Geometry check sheet. Reference: the model listing, model coordinates, mm. Give positions to 0.01 mm unless a question says otherwise; leave off trailing zeros. Write each loop counter-clockwise with the first axis right and the second up, starting at its lowest first coordinate (ties: lowest second). Pieces come first, ordered by that corner, then holes. Notation, with made-up numbers: (36, 86.5) -> (66, 86.5) arc R18 ccw to (66, 114.5) -> close; hole circle Ø3 at (86, 73.5). An arc over 180 degrees is marked (long way). One line per item, written item: value.
from build123d import *

# Parameters (mm, degrees)
ESQUISSE1_R        = 11
ESQUISSE1_R_2      = 1.65
ESQUISSE1_R_3      = 3
BOSS_EXTRU_1_DEPTH = 4
CHANFREIN1_SIZE    = 0.5


with BuildPart() as part:
    # Esquisse1 → Boss.-Extru.1 (new body)
    with BuildSketch(Plane(origin=(0, 0, 0), x_dir=(1, 0, 0), z_dir=(0, 1, 0))):
        with Locations(Location((0, 0, 0), (0, 0, 270))):
            Circle(ESQUISSE1_R)
        with Locations(Location((0, 7, 0), (0, 0, 270))):
            Circle(ESQUISSE1_R_2, mode=Mode.SUBTRACT)
        with Locations(Location((7, 0, 0), (0, 0, 270))):
            Circle(ESQUISSE1_R_2, mode=Mode.SUBTRACT)
        with Locations(Location((0, -7, 0), (0, 0, 270))):
            Circle(ESQUISSE1_R_2, mode=Mode.SUBTRACT)
        with Locations(Location((-7, 0, 0), (0, 0, 270))):
            Circle(ESQUISSE1_R_2, mode=Mode.SUBTRACT)
        with Locations(Location((0, 0, 0), (0, 0, 270))):
            Circle(ESQUISSE1_R_3, mode=Mode.SUBTRACT)
    extrude(amount=BOSS_EXTRU_1_DEPTH)

    # Chanfrein1
    chanfrein1_edges = [part.edges().sort_by_distance(p)[0] for p in [
        (0, 0, -11),
        (0, 4, -11),
    ]]
    chamfer(chanfrein1_edges, length=CHANFREIN1_SIZE)


solid = part.part
1) Sectioned sample at B-B on z = 0. Record the cut outline in (x, y).
Verdict:
outline: (-11, 0.5) -> (-10.5, 0) -> (-8.65, 0) -> (-8.65, 4) -> (-10.5, 4) -> (-11, 3.5) -> close; (-5.35, 0) -> (-3, 0) -> (-3, 4) -> (-5.35, 4) -> close; (3, 0) -> (5.35, 0) -> (5.35, 4) -> (3, 4) -> close; (8.65, 0) -> (10.5, 0) -> (11, 0.5) -> (11, 3.5) -> (10.5, 4) -> (8.65, 4) -> close
2) Depth check by flat-ended pin: pin 1 Ø3 at (x, z) = (0, 7) entering from +Y; pin 2 Ø1.5 at (y, z) = (1, 6) entering from +X; pin 3 Ø2 at (x, y) = (-3.5, 1) entering from +Z; pin 4 Ø1 at (y, z) = (2, -7.5) entering from -X. Enter the tip coordinate at first touch or a pass-through.
Verdict:
pin 1: through
pin 2: x = 9.67
pin 3: z = 10.71
pin 4: x = -8.49
3) Scan lines: probe 1 along X at (y, z) = (1.15, 0); probe 2 along Z at (x, y) = (-6, 0.75); probe 3 along X at (y, z) = (0.9, 7). Record each from-to range of solid material in increasing order.
Verdict:
probe 1: -11 to -8.65, -5.35 to -3, 3 to 5.35, 8.65 to 11
probe 2: -9.22 to -1.31, 1.31 to 9.22
probe 3: -8.49 to -1.65, 1.65 to 8.49
4) Sectioned sample at C-C on y = 2.7. Record the cut outline in (x, z).
Verdict:
outline: circle Ø22 at (0, 0); hole circle Ø3.3 at (-7, 0); hole circle Ø6 at (0, 0); hole circle Ø3.3 at (0, -7); hole circle Ø3.3 at (0, 7); hole circle Ø3.3 at (7, 0)
5) Mould release check, pull along X, two halves, no side actions. Record for faces 1 (the cylindrical face through (5.4, 2, -0.4)), 2 (the cylindrical face through (-8, 1.97, -1.31)), 3 (the cylindrical face through (-10.74, 1.98, -2.38)), 4 (the flat face through (2.5, 0, 2.2)): released by +X, released by -X, zero draft, split by the parting line, or undercut.
Verdict:
face 1: undercut
face 2: undercut
face 3: split by the parting line
face 4: zero draft
6) Sectioned sample at A-A on x = 0. Record the cut outline in (y, z).
Verdict:
outline: (0, -10.5) -> (0.5, -11) -> (3.5, -11) -> (4, -10.5) -> (4, -8.65) -> (0, -8.65) -> close; (0, -5.35) -> (4, -5.35) -> (4, -3) -> (0, -3) -> close; (0, 3) -> (4, 3) -> (4, 5.35) -> (0, 5.35) -> close; (0, 8.65) -> (4, 8.65) -> (4, 10.5) -> (3.5, 11) -> (0.5, 11) -> (0, 10.5) -> close
